Model file for the job. Use its own axes, mm. A direction names the side the tool comes from. Give positions to 0.01 mm unless a question says otherwise; leave off trailing zeros. Loops run counter-clockwise (first coordinate to the right, second up) from the corner with the lowest first, then second, coordinate; pieces in that order, holes last. Notation, with made-up numbers: (35, -16.75) - (55, -16.75) arc R15 ccw to (55, 9.25) - close; hole circle Ø10 at (74, 58). An arc over 180 degrees is marked (long way). Answer as CSV lines item,"result". Start each with the question number.
Item 1: Tool access for faces 4 (the cylindrical face through (25.12, 2.46, -43.23)), 5 (the flat face through (-61.166, 2.465, 35.057)), 6 (the flat face through (26.91, 2.535, -24.197)), 7 (the flat face through (61.166, 2.465, -35.057)), 8 (the cylindrical face through (-8.618, 5.107, -20.784)): list every direction of +Z, -Z, +X, -X, +Y, -Y with a clear straight run to the whole face (end or side of a thin tool).
Item 2: Pull direction Z, two halves, no side cores. Call faces 1 (the cylindrical face through (-25.12, 2.46, 43.23)), 2 (the cylindrical face through (-50, 2, 0)), 3 (the flat face through (30, 5, 15)): pulls with the +Z half, pulls with the -Z half, needs draft (parallel to the pull), parting line crosses it, or undercut.
Item 3: Saw through at A-A on z = 60. Give the cut face in (x, y).
Item 4: Pin check, flat tips, straight feed: pin 1 (1.5 mm diameter, centred on y = 4, z = -36.5, fed in from +X); pin 2 (2.5 mm diameter, centred on y = 1.5, z = -56, fed in from +X); pin 3 (5.5 mm diameter, centred on y = 1.5, z = -36, fed in from -X). Stop position of each tip, or through.
Item 5: Drill centre lines: L1, parallel to Z at x = -24, y = 2; L2, parallel to Z at x = 25.5, y = 2.5; L3, parallel to Y at x = -2, z = 49. Where is each one in solid material? Low to high. Write a range as from..to.
from build123d import *

# Parameters (mm, degrees)
BOSS_EXTRUDE1_DEPTH = 5
CIRPATTERN1_COUNT   = 3
CIRPATTERN1_ANGLE   = 120
SKETCH8_R           = 22.5
BOSS_EXTRUDE4_DEPTH = 10
SKETCH11_R          = 22.5
CUT_EXTRUDE4_DEPTH  = 11.7
SKETCH12_R          = 4
CUT_EXTRUDE5_DEPTH  = 3.3
SKETCH14_R          = 3.65
CUT_EXTRUDE7_DEPTH  = 100.784323589
CIRPATTERN2_COUNT   = 6
CUT_EXTRUDE9_DEPTH  = 15
SKETCH16_R          = 2.4
SKETCH16_R_2        = 3.65
CUT_EXTRUDE10_DEPTH = 2.46
CIRPATTERN3_COUNT   = 6
SKETCH17_R          = 4
SKETCH17_R_2        = 3.65
BOSS_EXTRUDE5_DEPTH = 3.3
CUT_EXTRUDE11_START = -2.1
SKETCH18_R          = 2.4
SKETCH18_R_2        = 3.65
CUT_EXTRUDE11_DEPTH = 2.1
BOSS_EXTRUDE6_START = 1.34
SKETCH21_R          = 22.5
BOSS_EXTRUDE6_DEPTH = 1.34
CUT_EXTRUDE12_START = -10.34
SKETCH22_R          = 3.65
CUT_EXTRUDE12_DEPTH = 10.34


# Read off the part's stored shape, not the designer's step: Boundary2
with BuildPart() as part:
    # Sketch1 → Boss-Extrude1 (new body)
    with BuildSketch(Plane(origin=(0, 0, 0), x_dir=(1, 0, 0), z_dir=(0, 1, 0))):
        with BuildLine():
            ThreePointArc((-15.9, 47.404535648), (-50, 0), (-15.9, -47.404535648))
            Line((-15.9, -47.404535648), (-15.9, 47.404535648))
        make_face()
        with BuildLine():
            ThreePointArc((-15.9, -47.404535648), (0, -50), (15.9, -47.404535648))
            Line((15.9, -47.404535648), (15.9, 47.404535648))
            ThreePointArc((15.9, 47.404535648), (0, 50), (-15.9, 47.404535648))
            Line((-15.9, 47.404535648), (-15.9, -47.404535648))
        make_face()
        with BuildLine():
            Line((-15.9, -70.5), (15.9, -70.5))
            Line((15.9, -70.5), (15.9, -47.404535648))
            ThreePointArc((15.9, -47.404535648), (0, -50), (-15.9, -47.404535648))
            Line((-15.9, -47.404535648), (-15.9, -70.5))
        make_face()
        with BuildLine():
            ThreePointArc((-15.9, 47.404535648), (0, 50), (15.9, 47.404535648))
            Line((15.9, 47.404535648), (15.9, 70.5))
            Line((15.9, 70.5), (-15.9, 70.5))
            Line((-15.9, 70.5), (-15.9, 47.404535648))
        make_face()
        with BuildLine():
            Line((15.9, 47.404535648), (15.9, -47.404535648))
            ThreePointArc((15.9, -47.404535648), (40.589407485, -29.197602641), (50, 0))
            ThreePointArc((50, 0), (40.589407485, 29.197602641), (15.9, 47.404535648))
        make_face()
    boss_extrude1 = extrude(amount=BOSS_EXTRUDE1_DEPTH)

    # CirPattern1: Boss-Extrude1 ×3 about axis
    cirpattern1_axis = Axis((0, 0, 0), (0, 1, 0))
    for i in range(1, CIRPATTERN1_COUNT):
        add(boss_extrude1.rotate(cirpattern1_axis, i * CIRPATTERN1_ANGLE / (CIRPATTERN1_COUNT - 1)))

    # Sketch8 → Boss-Extrude4 (add)
    with BuildSketch(Plane(origin=(0, 5, 0), x_dir=(1, 0, 0), z_dir=(0, 1, 0))):
        with Locations(Location((0, 0, 0), (0, 0, 270))):
            Circle(SKETCH8_R)
    extrude(amount=BOSS_EXTRUDE4_DEPTH)

    # Boundary2 outline → Boundary2 (revolve)
    with BuildSketch(Plane.XY):
        Polygon((32.5, 5), (22.499998072, 15.000001928), (22.5, 5), align=None)
    revolve(axis=Axis((0, 0, 0), (0, 1, 0)))

    # Sketch11 → Cut-Extrude4 (cut)
    with BuildSketch(Plane.XZ):
        with Locations(Location((0, 0, 0), (0, 0, 270))):
            Circle(SKETCH11_R)
    extrude(amount=-CUT_EXTRUDE4_DEPTH, mode=Mode.SUBTRACT)

    # Sketch12 → Cut-Extrude5 (cut)
    with BuildSketch(Plane.XZ.offset(-11.7)):
        with Locations(Location((0, 0, 0), (0, 0, 270))):
            Circle(SKETCH12_R)
    extrude(amount=-CUT_EXTRUDE5_DEPTH, mode=Mode.SUBTRACT)

    # Sketch14 → Cut-Extrude7 (cut, through all)
    with BuildSketch(Plane(origin=(0, 0, 0), x_dir=(-1, 0, 0), z_dir=(0, -1, 0))):
        with Locations(Location((5.17, -60, 0), (0, 0, 90))):
            Circle(SKETCH14_R)
    cut_extrude7 = extrude(amount=-CUT_EXTRUDE7_DEPTH, mode=Mode.SUBTRACT)

    # CirPattern2: Cut-Extrude7 ×6 about axis
    cirpattern2_axis = Axis((0, 0, 0), (0, 1, 0))
    for i in range(1, CIRPATTERN2_COUNT):
        add(cut_extrude7.rotate(cirpattern2_axis, i * 360 / CIRPATTERN2_COUNT), mode=Mode.SUBTRACT)

    # Sketch15 → Cut-Extrude9 (cut)
    with BuildSketch(Plane(origin=(0, 5, 0), x_dir=(1, 0, 0), z_dir=(0, 1, 0))):
        with BuildLine():
            Line((-37.776643972, 13.150101528), (-31.136127875, 9.316197772))
            ThreePointArc((-31.136127875, 9.316197772), (-32.5, 0), (-31.136127875, -9.316197772))
            Line((-31.136127875, -9.316197772), (-37.776643972, -13.150101528))
            ThreePointArc((-37.776643972, -13.150101528), (-40, 0), (-37.776643972, 13.150101528))
        make_face()
        with BuildLine():
            Line((-30.276643972, 26.140482585), (-23.636127875, 22.306578829))
            ThreePointArc((-23.636127875, 22.306578829), (-16.25, 28.145825623), (-7.5, 31.622776602))
            Line((-7.5, 31.622776602), (-7.5, 39.290584114))
            ThreePointArc((-7.5, 39.290584114), (-20, 34.641016151), (-30.276643972, 26.140482585))
        make_face()
        with BuildLine():
            Line((7.5, 39.290584114), (7.5, 31.622776602))
            ThreePointArc((7.5, 31.622776602), (16.25, 28.145825623), (23.636127875, 22.306578829))
            Line((23.636127875, 22.306578829), (30.276643972, 26.140482585))
            ThreePointArc((30.276643972, 26.140482585), (20, 34.641016151), (7.5, 39.290584114))
        make_face()
        with BuildLine():
            Line((37.776643972, 13.150101528), (31.136127875, 9.316197772))
            ThreePointArc((31.136127875, 9.316197772), (32.5, 0), (31.136127875, -9.316197772))
            Line((31.136127875, -9.316197772), (37.776643972, -13.150101528))
            ThreePointArc((37.776643972, -13.150101528), (40, 0), (37.776643972, 13.150101528))
        make_face()
        with BuildLine():
            Line((30.276643972, -26.140482585), (23.636127875, -22.306578829))
            ThreePointArc((23.636127875, -22.306578829), (16.25, -28.145825623), (7.5, -31.622776602))
            Line((7.5, -31.622776602), (7.5, -39.290584114))
            ThreePointArc((7.5, -39.290584114), (20, -34.641016151), (30.276643972, -26.140482585))
        make_face()
        with BuildLine():
            Line((-7.5, -39.290584114), (-7.5, -31.622776602))
            ThreePointArc((-7.5, -31.622776602), (-16.25, -28.145825623), (-23.636127875, -22.306578829))
            Line((-23.636127875, -22.306578829), (-30.276643972, -26.140482585))
            ThreePointArc((-30.276643972, -26.140482585), (-20, -34.641016151), (-7.5, -39.290584114))
        make_face()
    extrude(amount=-CUT_EXTRUDE9_DEPTH, mode=Mode.SUBTRACT)

    # Sketch16 → Cut-Extrude10 (cut)
    with BuildSketch(Plane.XZ):
        with Locations((-10.93, -60)):
            Circle(SKETCH16_R)
        with BuildLine():
            Line((4.886614907, -56.361017603), (-11.116335404, -57.607244451))
            ThreePointArc((-11.116335404, -57.607244451), (-9.300154144, -58.238295574), (-8.53, -60))
            ThreePointArc((-8.53, -60), (-9.300154144, -61.761704426), (-11.116335404, -62.392755549))
            Line((-11.116335404, -62.392755549), (4.886614907, -63.638982397))
            ThreePointArc((4.886614907, -63.638982397), (1.52, -60), (4.886614907, -56.361017603))
        make_face()
        with Locations(Location((5.17, -60, 0), (0, 0, 94.452911391))):
            Circle(SKETCH16_R_2)
    cut_extrude10 = extrude(amount=-CUT_EXTRUDE10_DEPTH, mode=Mode.SUBTRACT)

    # CirPattern3: Cut-Extrude10 ×6 about axis
    cirpattern3_axis = Axis((0, 0, 0), (0, 1, 0))
    for i in range(1, CIRPATTERN3_COUNT):
        add(cut_extrude10.rotate(cirpattern3_axis, i * 360 / CIRPATTERN3_COUNT), mode=Mode.SUBTRACT)

    # Sketch17 → Boss-Extrude5 (add)
    with BuildSketch(Plane.XZ.offset(-11.7)):
        Circle(SKETCH17_R)
        with Locations(Location((0, 0, 0), (0, 0, 270))):
            Circle(SKETCH17_R_2, mode=Mode.SUBTRACT)
    extrude(amount=-BOSS_EXTRUDE5_DEPTH)

    # Sketch18 → Cut-Extrude11 (cut)
    with BuildSketch(Plane(origin=(0, 15, 0), x_dir=(1, 0, 0), z_dir=(0, 1, 0)).offset(CUT_EXTRUDE11_START)):
        with BuildLine():
            Line((-16.286335404, -2.392755549), (-0.283385093, -3.638982397))
            ThreePointArc((-0.283385093, -3.638982397), (-3.65, 0), (-0.283385093, 3.638982397))
            Line((-0.283385093, 3.638982397), (-16.286335404, 2.392755549))
            ThreePointArc((-16.286335404, 2.392755549), (-14.470154144, 1.761704426), (-13.7, 0))
            ThreePointArc((-13.7, 0), (-14.470154144, -1.761704426), (-16.286335404, -2.392755549))
        make_face()
        with Locations((-16.1, 0)):
            Circle(SKETCH18_R)
        with Locations(Location((0, 0, 0), (0, 0, 90))):
            Circle(SKETCH18_R_2)
    extrude(amount=CUT_EXTRUDE11_DEPTH, mode=Mode.SUBTRACT)

    # Sketch21 → Boss-Extrude6 (add)
    with BuildSketch(Plane(origin=(0, 11.7, 0), x_dir=(-1, 0, 0), z_dir=(0, -1, 0)).offset(BOSS_EXTRUDE6_START)):
        with Locations(Location((0, 0, 0), (0, 0, 90))):
            Circle(SKETCH21_R)
    extrude(amount=-BOSS_EXTRUDE6_DEPTH)

    # Sketch22 → Cut-Extrude12 (cut)
    with BuildSketch(Plane(origin=(0, 15, 0), x_dir=(1, 0, 0), z_dir=(0, 1, 0)).offset(CUT_EXTRUDE12_START)):
        with Locations(Location((0, 0, 0), (0, 0, 90))):
            Circle(SKETCH22_R)
    extrude(amount=CUT_EXTRUDE12_DEPTH, mode=Mode.SUBTRACT)


solid = part.part
Responses:
1,face 4,"-Z, +Y, -Y"
1,face 5,"+Z, -X, +Y, -Y"
1,face 6,"+Y, -Y"
1,face 7,"-Z, +X, +Y, -Y"
1,face 8,"-Y"
2,face 1,"pulls with the +Z half"
2,face 2,"undercut"
2,face 3,"needs draft"
3,outline,"(-15.9, 0) - (-8.82, 0) - (-8.82, 5) - (-15.9, 5) - close; (-1.52, 2.46) - (13.33, 2.46) - (13.33, 0) - (15.9, 0) - (15.9, 5) - (-1.52, 5) - close"
4,pin 1,"x = 60.77"
4,pin 2,"x = 15.9"
4,pin 3,"x = -62.21"
5,L1,"-43.86..-32, -22.52..22.52, 32..43.86"
5,L2,"-43.01..-30.82, -23.38..23.38, 30.82..43.01"
5,L3,"0..5"
